from build123d import *

# Parameters (mm, degrees)
F1_DEPTH  = 6
F3_T      = -1.5
F4_R      = 1
F5_DEPTH  = 26
F6_W      = 9
F6_H      = 9
F7_DEPTH  = 3
F8_R      = 2
F8_R_2    = 1
F9_DEPTH  = 9
F11_DEPTH = 7.5
F12_DEPTH = 2.5
F14_DEPTH = 0.75


# Not quite as in the source:
# - a feature names something its author has since deleted; it is built from what else it names


with BuildPart() as f1:
    # F0 (on Top) → F1 (new body)
    with BuildSketch(Plane.XY):
        with BuildLine():
            Line((-65, 4.5), (-65, 3))
            Line((-65, 3), (-59, -6))
            Line((-59, -6), (0, -6))
            Line((0, -6), (0, 6))
            Line((0, 6), (-34.5, 6))
            Line((-34.5, 6), (-39.5, 0))
            Line((-39.5, 0), (-53, 0))
            Line((-53, 0), (-56, 4.5))
            ThreePointArc((-56, 4.5), (-60.5, 0), (-65, 4.5))
        make_face()
        with BuildLine():
            ThreePointArc((-64.7426406871, 6), (-64.9351935184, 5.2609589043), (-65, 4.5))
            ThreePointArc((-65, 4.5), (-60.5, 0), (-56, 4.5))
            ThreePointArc((-56, 4.5), (-56.0648064816, 5.2609589043), (-56.2573593129, 6))
            Line((-56.2573593129, 6), (-64.7426406871, 6))
        make_face()
        with BuildLine():
            ThreePointArc((-56.2573593129, 6), (-60.5, 9), (-64.7426406871, 6))
            Line((-64.7426406871, 6), (-56.2573593129, 6))
        make_face()
    extrude(amount=F1_DEPTH)

    # F2: F1 across plane


with BuildPart() as f1_1:
    add(f1.part)
    add(f1.part.mirror(Plane.YZ))

    # F3
    f3_openings = [f1_1.faces().sort_by_distance(p)[0] for p in [
        (0, -0.200074, 6),
    ]]
    offset(amount=F3_T, openings=f3_openings, kind=Kind.INTERSECTION)

    # F4 (on face) → F5 (cut)
    with BuildSketch(Plane.XY.offset(1.5)):
        with BuildLine():
            ThreePointArc((-57.5283708886, 4.0883928763), (-57.5071011265, 4.2937081366), (-57.5, 4.5))
            ThreePointArc((-57.5, 4.5), (-60.5, 7.5), (-63.5, 4.5))
            ThreePointArc((-63.5, 4.5), (-60.7062918634, 1.5071011265), (-57.5283708886, 4.0883928763))
        make_face()
        with Locations((-60.5, 4.5)):
            Circle(F4_R, mode=Mode.SUBTRACT)
    extrude(amount=F5_DEPTH, mode=Mode.SUBTRACT)

    # F6 (on face) → F7 (join)
    with BuildSketch(Plane.XY.offset(1.5)):
        Rectangle(F6_W, F6_H)
    extrude(amount=F7_DEPTH)

    # F8 (on face) → F9 (join)
    with BuildSketch(Plane.XY.offset(4.5)):
        with Locations((0, 2)):
            Circle(F8_R)
        with Locations((0, 2)):
            Circle(F8_R_2, mode=Mode.SUBTRACT)
    extrude(amount=F9_DEPTH)

    # F10 (on face) → F11 (join)
    with BuildSketch(Plane(origin=(0, 0, 0), x_dir=(1, 0, 0), z_dir=(0, 0, -1))):
        Polygon((4.35, 6), (-4.35, 6), (-4.35, -6), (-2.85, -6), (-2.85, 4.5), (2.85, 4.5), (2.85, -6), (4.35, -6), align=None)
    extrude(amount=F11_DEPTH)

    # F12 (cut): a face of the model
    f12_faces = [f1_1.faces().sort_by_distance(p)[0] for p in [
        (0, 0.75, 0),
    ]]
    extrude(f12_faces, amount=-F12_DEPTH, mode=Mode.SUBTRACT)

    # F13 (on Front) → F14 (join, symmetric)
    with BuildSketch(Plane.XZ):
        Polygon((4.35, 0), (4.35, -4), (14.85, -2.5), (14.85, 0), align=None)
        Polygon((-14.85, -2.5), (-4.35, -4), (-4.35, 0), (-14.85, 0), align=None)
    extrude(amount=F14_DEPTH, both=True)


solid = f1_1.part
Geometry check sheet. Reference: the model listing, model coordinates, mm. A direction names the side the tool comes from. Coordinates: 2 decimals unless noted, no trailing zeros. Loops run counter-clockwise (first coordinate to the right, second up) from the corner with the lowest first, then second, coordinate; pieces in that order, holes last. Notation, with made-up numbers: (-34, -3) - (12, -3) arc R14 cw to (12, 20) - close; hole circle Ø7 at (-38, -25). An arc over 180 degrees is marked (long way). Use one line per item in the form item = value. Start each with the question number.
Item 1: Section check A-A, the plane x = -32.5. Enter the section's corners in (y, z), and give its area (3 significant figures).
Item 2: Thickness scan on probe 1 along Y at (x, z) = (-33, 5.25); probe 2 along Y at (x, z) = (0, 11.25); probe 3 along X at (y, z) = (-2.5, -5.75). Record the ranges inside material, lowest first.
Item 3: Section check B-B, the plane z = -5.5. Enter the section's corners in (x, y), and give its area (4 significant figures).
Item 4: Tool access check on faces 1 (the face through (0, -4.5, -2)), 2 (the face through (-4.35, 0, -5)), 3 (the face through (-4.5, 0, 3)). Record the directions out of +Z, -Z, +X, -X, +Y, -Y that give a thin tool (end or side, any length) a straight path to the whole face; none if there is none.
Item 5: Section check C-C, the plane y = -3.25. Enter the section's corners in (x, z), and give its area (3 significant figures).
Item 6: Gauge pin test, flat ends, axial feed: pin 1 (6 mm diameter, centred on y = -0.5, z = -3.5, fed in from +X); pin 2 (2.5 mm diameter, centred on y = 0.5, z = 2.5, fed in from +X); pin 3 (4 mm diameter, centred on x = 12.5, z = -3.5, fed in from +Y). Record the tip position at first contact, or that the pin passes through.
Item 7: Mould release check, pull along Y, two halves, no side actions. Record for faces 4 (the face through (-27, 0, 1.5)), 5 (the face through (1, -6, 2)), 6 (the face through (0, -5, 6)): +Y half, -Y half, draft (parallel to the pull), parting line (faces both ways), or undercut.
Computed:
q1.outline = (-6, 0) - (6, 0) - (6, 6) - (4.5, 6) - (4.5, 1.5) - (-4.5, 1.5) - (-4.5, 6) - (-6, 6) - close
q1.area = 31.5 mm2
q2.probe_1 = -6 to -4.5, 4.5 to 6
q2.probe_2 = 0 to 1, 3 to 4
q2.probe_3 = -4.35 to -2.85, 2.85 to 4.35
q3.outline = (-4.35, -6) - (4.35, -6) - (4.35, 6) - (2.85, 6) - (2.85, -4.5) - (-2.85, -4.5) - (-2.85, 6) - (-4.35, 6) - close
q3.area = 44.55 mm2
q4.face_1 = -Z, +Y
q4.face_2 = -Z, -X
q4.face_3 = +Z
q5.outline = (-60.83, 0) - (-4.35, 0) - (-4.35, -7.5) - (-2.85, -7.5) - (-2.85, 2.5) - (2.85, 2.5) - (2.85, -7.5) - (4.35, -7.5) - (4.35, 0) - (60.83, 0) - (60.83, 6) - (59.03, 6) - (59.03, 1.5) - (4.5, 1.5) - (4.5, 4.5) - (-4.5, 4.5) - (-4.5, 1.5) - (-59.03, 1.5) - (-59.03, 6) - (-60.83, 6) - close
q5.area = 234 mm2
q6.pin_1 = 14.85
q6.pin_2 = 64.17
q6.pin_3 = 0.75
q7.face_4 = undercut
q7.face_5 = -Y half
q7.face_6 = draft
